from build123d import *

# Parameters (mm, degrees)
SKETCH1_R           = 2.5
BOSS_EXTRUDE1_DEPTH = 2


with BuildPart() as part:
    # Sketch1 → Boss-Extrude1 (new body)
    with BuildSketch(Plane.XY):
        with BuildLine():
            Line((-85, 33.5), (-85, -33.5))
            Line((-85, -33.5), (85, -33.5))
            Line((85, -33.5), (85, 33.5))
            Line((85, 33.5), (-26.703847577, 33.5))
            ThreePointArc((-26.703847577, 33.5), (-31.9, 30.5), (-37.096152423, 33.5))
            Line((-37.096152423, 33.5), (-85, 33.5))
        make_face()
        with Locations((-68.3, -21.5)):
            Circle(SKETCH1_R, mode=Mode.SUBTRACT)
        with Locations((-74.1, 1.5)):
            Circle(SKETCH1_R, mode=Mode.SUBTRACT)
        with Locations((76.2, -22)):
            Circle(SKETCH1_R, mode=Mode.SUBTRACT)
        with Locations((18.7, -8.7)):
            Circle(SKETCH1_R, mode=Mode.SUBTRACT)
        with Locations((78.2, -0.1)):
            Circle(SKETCH1_R, mode=Mode.SUBTRACT)
        with Locations((-65.3, 20)):
            Circle(SKETCH1_R, mode=Mode.SUBTRACT)
        with Locations((8.2, 8.3)):
            Circle(SKETCH1_R, mode=Mode.SUBTRACT)
        with Locations((28.1, 9)):
            Circle(SKETCH1_R, mode=Mode.SUBTRACT)
        with Locations((73.2, 22.3)):
            Circle(SKETCH1_R, mode=Mode.SUBTRACT)
    extrude(amount=BOSS_EXTRUDE1_DEPTH)


solid = part.part
Geometry check sheet. Reference: the model listing, model coordinates, mm. Round coordinates to 2 decimals unless told otherwise and drop trailing zeros. Write each loop counter-clockwise with the first axis right and the second up, starting at its lowest first coordinate (ties: lowest second). Pieces come first, ordered by that corner, then holes. Notation, with made-up numbers: (-18.5, 37.25) -> (3.5, 37.25) arc R19 cw to (3.5, 50.25) -> close; hole circle Ø8 at (52.5, -21). An arc over 180 degrees is marked (long way). One line per item, written item: value. Start each with the question number.
(1) Cross-section at A-A, the plane z = 0.7. Give the number of separate pieces and of enclosed holes in the cut face, and give its area (3 significant figures).
(2) Draft check along Y on faces 1 (the flat face through (-1, 0, 2)), 2 (the cylindrical face through (-31.8, 30.5, 1)), 3 (the cylindrical face through (29.25, 6.78, 0.99)), 4 (the cylindrical face through (-76.6, 1.6, 1)). Enter one of: +Y half, -Y half, draft (parallel to the pull), parting line (faces both ways), or undercut.
(3) Scan lines: line 1 (Y direction, x = 19, z = 0.3); line 2 (Y direction, x = 78.5, z = 1.95); line 3 (Y direction, x = 78.2, z = 1.05). Record each from-to range of solid material in increasing order. Write a range as [from, to].
(4) Cross-section at C-C, the plane y = -8.7. Record the cut outline in (x, z).
(5) Cross-section at B-B, the plane x = -74.1. Record the cut outline in (y, z).
(6) Go/stop test with a flat-tipped pin: pin 1 Ø1 at (x, z) = (-33.5, 0.5) entering from +Y. Record where the tip stops, or that it passes through.
Answer:
1. separate pieces: 1
1. enclosed holes: 9
1. area: 11,200 mm²
2. face 1: draft
2. face 2: +Y half
2. face 3: undercut
2. face 4: undercut
3. line 1: [-33.5, -11.18], [-6.22, 33.5]
3. line 2: [-33.5, -22.98], [-21.02, -2.58], [2.38, 33.5]
3. line 3: [-33.5, -23.5], [-20.5, -2.6], [2.4, 33.5]
4. outline: (-85, 0) -> (16.2, 0) -> (16.2, 2) -> (-85, 2) -> close; (21.2, 0) -> (85, 0) -> (85, 2) -> (21.2, 2) -> close
5. outline: (-33.5, 0) -> (-1, 0) -> (-1, 2) -> (-33.5, 2) -> close; (4, 0) -> (33.5, 0) -> (33.5, 2) -> (4, 2) -> close
6. pin 1: y = 30.88
